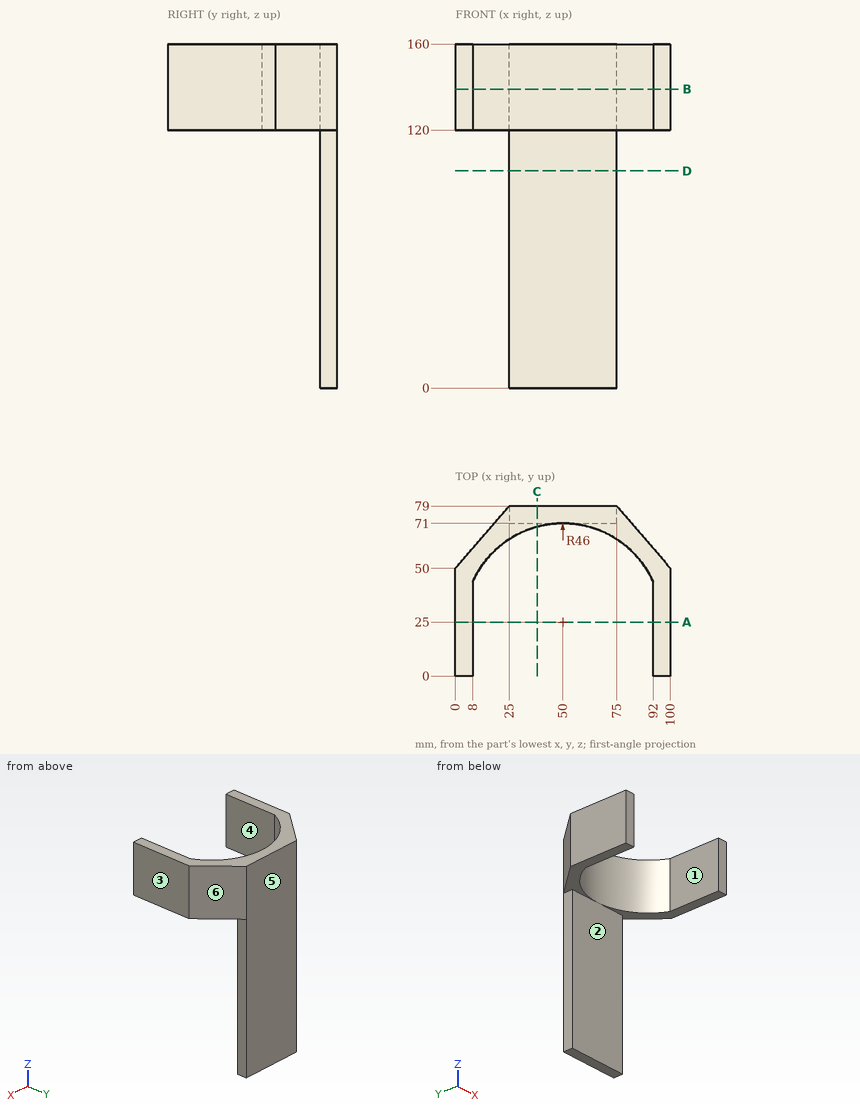
Part print with two shaded views. Sizes in mm from the minimum x, y, z corner. A direction names the side the tool comes from. Round coordinates to 2 decimals unless told otherwise and drop trailing zeros. Loops run counter-clockwise (first coordinate to the right, second up) from the corner with the lowest first, then second, coordinate; pieces in that order, holes last.
1. Drill centre lines: line 1 along X through (y, z) = (31, 121); line 2 along Y through (x, z) = (47, 76); line 3 along Z through (x, y) = (22.5, 66). Where is each one in solid material? Low to high.
Solutions:
line 1: x = 0 to 8, 92 to 100
line 2: y = 71 to 79
line 3: z = 120 to 160
2. 3-axis set-ups, long thin cutter, end or side, ignore diameter. For the marked faces 1, 2 and 3: which of +Z, -Z, +X, -X, +Y, -Y reach the whole face in a straight line?
Solutions:
face 1: +Z, -Z, -Y
face 2: -Z, +X, -X, -Y
face 3: +Z, -Z, +X, +Y, -Y
3. Slice it at B-B (z = 139). Give the cut face in (x, y), and give its area (3 significant figures).
Solutions:
outline: (0, 0) - (8, 0) - (8, 43.76) arc R46 cw to (92, 43.76) - (92, 0) - (100, 0) - (100, 50) - (75, 79) - (25, 79) - (0, 50) - close
area: 1,850 mm2
4. Slice it at A-A (y = 25). Give the cut face in (x, z).
Solutions:
outline: (0, 120) - (8, 120) - (8, 160) - (0, 160) - close; (92, 120) - (100, 120) - (100, 160) - (92, 160) - close
5. Flat gauge pins, fed straight in: pin 1 (10 mm diameter, centred on y = 70.5, z = 120.5, fed in from +X); pin 2 (4 mm diameter, centred on y = 73, z = 78, fed in from -X); pin 3 (9 mm diameter, centred on y = 76, z = 86, fed in from +X). Where does each tip first touch, or does it go through?
Solutions:
pin 1: stops at x = 86.64
pin 2: stops at x = 25
pin 3: stops at x = 75
6. Slice it at C-C (x = 38). Give the cut face in (y, z), and give its area (3 significant figures).
Solutions:
outline: (69.41, 120) - (71, 120) - (71, 0) - (79, 0) - (79, 160) - (69.41, 160) - close
area: 1,340 mm2
7. Slice it at D-D (z = 101). Give the cut face in (x, y).
Solutions:
outline: (25, 71) - (75, 71) - (75, 79) - (25, 79) - close
8. Two-plate mould, pull along X, no slides. Class the marked faces 4, 5 and 6: pulls with the +X half, pulls with the -X half, needs draft (parallel to the pull), parting line crosses it, or undercut.
Solutions:
face 4: undercut
face 5: needs draft
face 6: pulls with the +X half
